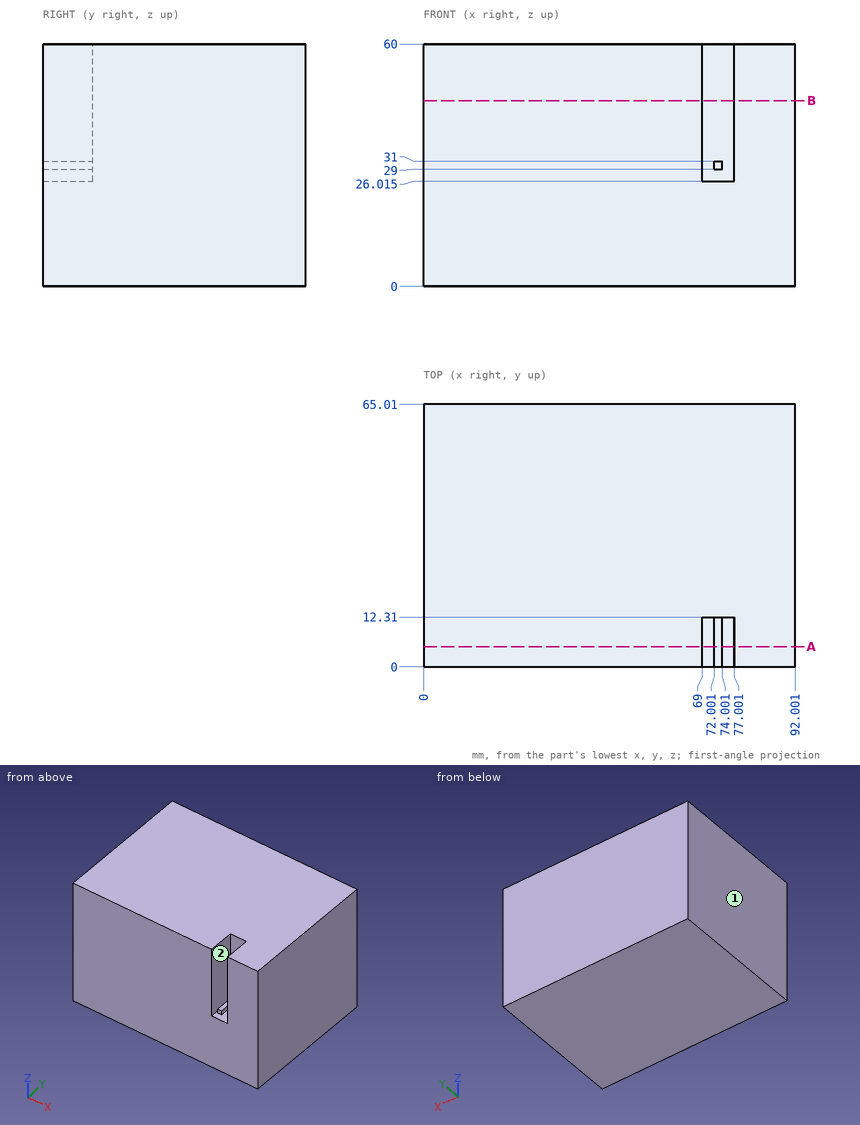
Could you check a few things on this drawing? It's one solid part, dimensions in mm from its lowest x, y, z. A direction names the side the tool comes from. Round coordinates to 2 decimals unless told otherwise and drop trailing zeros. Write each loop counter-clockwise with the first axis right and the second up, starting at its lowest first coordinate (ties: lowest second). Pieces come first, ordered by that corner, then holes.
Q1. Which directions (+Z, -Z, +X, -X, +Y, -Y) give clear straight access to the entire face, cutting with the end or side of a thin tool? Please do the marked faces 1 and 2.
Q2. If we section it at A-A on y = 5: Write out the boundary of the cut face in (x, z) (1 decimal), plus the area to 3 significant figures.
Q3. Please list where these lines run through material, in increasing order: probe 1 along X at (y, z) = (11, 54); probe 2 along Y at (x, z) = (73, 55).
Q4. If we section it at B-B on z = 46: Write out the boundary of the cut face in (x, y).
Q5. Will these pins go through, and if not, where does the flat tip stop? P1, Ø2.5, axis at x = 73.5, z = 48, coming from the -Y side; P2, Ø2, axis at x = 73.5, y = 7.5, coming from the +Z side.
Answer below:
1. face 1: +Z, -Z, -X, +Y, -Y
1. face 2: +Z, -Y
2. outline: (0, 0) - (92, 0) - (92, 60) - (77, 60) - (77, 26) - (69, 26) - (69, 60) - (0, 60) - close; (72, 29) - (74, 29) - (74, 31) - (72, 31) - close
2. area: 5,250 mm2
3. probe 1: x = 0 to 69, 77 to 92
3. probe 2: y = 12.31 to 65.01
4. outline: (0, 0) - (69, 0) - (69, 12.31) - (77, 12.31) - (77, 0) - (92, 0) - (92, 65.01) - (0, 65.01) - close
5. P1: stops at y = 12.31
5. P2: stops at z = 31
